```python
from build123d import *

# Parameters (mm, degrees)
EXTRUDE1_DEPTH  = 160
LPATTERN1_COUNT = 3
LPATTERN1_PITCH = 60


with BuildPart() as part:
    # Sketch1 → Extrude1 (new body)
    with BuildSketch(Plane(origin=(-20, 0, 0), x_dir=(1, 0, 0), z_dir=(0, 0, 1))):
        with BuildLine():
            Line((12.5, 0.69999271), (13.199992786, 0))
            Line((13.199992786, 0), (26.800007214, 0))
            Line((26.800007214, 0), (27.5, 0.69999271))
            Line((27.5, 0.69999271), (27.5, 4.2000246))
            Line((27.5, 4.2000246), (24.8000183, 6.9000063))
            Line((24.8000183, 6.9000063), (24.8000183, 8.8400054))
            Line((24.8000183, 8.8400054), (25.755946813, 9.794179118))
            ThreePointArc((25.755946813, 9.794179118), (26.198484624, 10.690600567), (27.09432569, 11.13431209))
            Line((27.09432569, 11.13431209), (27.5, 11.5399866))
            Line((27.5, 11.5399866), (27.5, 12.8500204))
            Line((27.5, 12.8500204), (27.09432569, 13.268442751))
            ThreePointArc((27.09432569, 13.268442751), (26.202460867, 13.706434947), (25.755946813, 14.594063938))
            Line((25.755946813, 14.594063938), (25.3500197, 15))
            Line((25.3500197, 15), (14.6499803, 15))
            Line((14.6499803, 15), (14.244053187, 14.594063938))
            ThreePointArc((14.244053187, 14.594063938), (13.797539133, 13.706434947), (12.90567431, 13.268442751))
            Line((12.90567431, 13.268442751), (12.5, 12.8500204))
            Line((12.5, 12.8500204), (12.5, 11.5399866))
            Line((12.5, 11.5399866), (12.90567431, 11.13431209))
            ThreePointArc((12.90567431, 11.13431209), (13.801515376, 10.690600567), (14.244053187, 9.794179118))
            Line((14.244053187, 9.794179118), (15.1999817, 8.8400054))
            Line((15.1999817, 8.8400054), (15.1999817, 6.9000063))
            Line((15.1999817, 6.9000063), (12.5, 4.2000246))
            Line((12.5, 4.2000246), (12.5, 0.69999271))
        make_face()
    extrude(amount=-EXTRUDE1_DEPTH)

    # Sketch2 → Cut-Revolve1 (revolve, cut)
    with BuildSketch(Plane(origin=(0, 0, 0), x_dir=(0, 0, -1), z_dir=(1, 0, 0))):
        Polygon((20, 15), (23.75, 15), (23.75, 9.7), (22.25, 9.7), (22.25, 0), (20, 0), align=None)
    cut_revolve1 = revolve(axis=Axis((0, 0, -20), (0, 1, 0)), mode=Mode.SUBTRACT)

    # LPattern1: Cut-Revolve1 ×3
    with Locations(*[(0, 0, -i * LPATTERN1_PITCH) for i in range(1, LPATTERN1_COUNT)]):
        add(cut_revolve1, mode=Mode.SUBTRACT)


solid = part.part
```
Verification items for the finished model (mm, model axes). A direction names the side the tool comes from. Coordinates: 2 decimals unless noted, no trailing zeros. Order: outer loops, then holes, each group sorted by start corner. A loop starts at its lowest first (then second) coordinate and runs counter-clockwise, first axis right, second up. Notation, with made-up numbers: (34, -24.5) - (47, -24.5) arc R26 cw to (47, 6.5) - close; hole circle Ø4 at (17.5, 2.5). An arc over 180 degrees is marked (long way). Return JSON: item names as keys, results as strings.
(1) Thickness scan on line 1 along Z through (x, y) = (0, 13.1); line 2 along Z through (x, y) = (0, 6.75); line 3 along X through (y, z) = (7.25, -20). Record the ranges inside material, lowest first.
Filled sheet:
{"line 1": "z = -160 to -143.75, -136.25 to -83.75, -76.25 to -23.75, -16.25 to 0", "line 2": "z = -160 to -142.25, -137.75 to -82.25, -77.75 to -22.25, -17.75 to 0", "line 3": "x = -4.8 to -2.25, 2.25 to 4.8"}
(2) Section check A-A, the plane x = 0. Record the cut outline in (y, z).
Filled sheet:
{"outline": "(0, -160) - (15, -160) - (15, -143.75) - (9.7, -143.75) - (9.7, -142.25) - (0, -142.25) - close; (0, -137.75) - (9.7, -137.75) - (9.7, -136.25) - (15, -136.25) - (15, -83.75) - (9.7, -83.75) - (9.7, -82.25) - (0, -82.25) - close; (0, -77.75) - (9.7, -77.75) - (9.7, -76.25) - (15, -76.25) - (15, -23.75) - (9.7, -23.75) - (9.7, -22.25) - (0, -22.25) - close; (0, -17.75) - (9.7, -17.75) - (9.7, -16.25) - (15, -16.25) - (15, 0) - (0, 0) - close"}
(3) Go/stop test with flat-tipped pins: pin 1 (4 mm diameter, centred on x = 0.5, z = -21, fed in from +Y); pin 2 (3.5 mm diameter, centred on x = 0, z = -140, fed in from +Y); pin 3 (1.6 mm diameter, centred on y = 7.5, z = -111, fed in from -X); pin 4 (0.6 mm diameter, centred on y = 7.5, z = -68.5, fed in from +X). Record where each tip stops, or that it passes through.
Filled sheet:
{"pin 1": "stops at y = 9.7", "pin 2": "passes through", "pin 3": "stops at x = -5", "pin 4": "stops at x = 4.8"}
(4) Access from +Z, -Z, +X, -X, +Y, -Y to the whole of each face (thin tool, end or side, straight path). Record for faces 1 (the cylindrical face through (-0.676, 4.782, -22.146)), 2 (the flat face through (6.2, 5.5, -78.9)), 3 (the cylindrical face through (1.436, 12.313, -83.464)).
Filled sheet:
{"face 1": "+Y, -Y", "face 2": "+Z, -Z, +X", "face 3": "+Y"}
(5) Mould release check, pull along Y, two halves, no side actions. Record for faces 4 (the flat face through (4, 15, -79)), 5 (the flat face through (-6.1, 5.6, -78.9)), 6 (the cylindrical face through (-0.165, 12.313, -16.254)): pulls with the +Y half, pulls with the -Y half, needs draft (parallel to the pull), parting line crosses it, or undercut.
Filled sheet:
{"face 4": "pulls with the +Y half", "face 5": "undercut", "face 6": "needs draft"}
(6) Section check C-C, the plane z = -53.5. Record the cut outline in (x, y).
Filled sheet:
{"outline": "(-7.5, 0.7) - (-6.8, 0) - (6.8, 0) - (7.5, 0.7) - (7.5, 4.2) - (4.8, 6.9) - (4.8, 8.84) - (5.76, 9.79) arc R1.56 cw to (7.09, 11.13) - (7.5, 11.54) - (7.5, 12.85) - (7.09, 13.27) arc R1.56 cw to (5.76, 14.59) - (5.35, 15) - (-5.35, 15) - (-5.76, 14.59) arc R1.56 cw to (-7.09, 13.27) - (-7.5, 12.85) - (-7.5, 11.54) - (-7.09, 11.13) arc R1.56 cw to (-5.76, 9.79) - (-4.8, 8.84) - (-4.8, 6.9) - (-7.5, 4.2) - close"}
